CAD build for the part. Positions are in the model's coordinates, mm. Face numbers are marked on the shaded views. A direction names the side the tool comes from. Round coordinates to 2 decimals unless told otherwise and drop trailing zeros. Write each loop counter-clockwise with the first axis right and the second up, starting at its lowest first coordinate (ties: lowest second). Pieces come first, ordered by that corner, then holes. Notation, with made-up numbers: (26.25, -21.75) - (66.25, -21.75) arc R29 ccw to (66.25, 10.25) - close; hole circle Ø5 at (51.25, 4.25). An arc over 180 degrees is marked (long way). Answer in a Markdown table with one row per item.
Autodesk Inventor part; units mm, degrees
ref_plane "YZ Plane" through (0, 0, 0) normal (1, 0, 0) x (0, 1, 0)
ref_plane "XZ Plane" through (0, 0, 0) normal (0, 1, 0) x (-1, 0, 0)
ref_plane "XY Plane" through (0, 0, 0) normal (0, 0, 1) x (1, 0, 0)
sketch "Sketch1" plane through (0, 0, 0) normal (0, 1, 0) x (-1, 0, 0)
  line L0 (10.6592, 57.15) -> (-7.8828, 57.15)
  line L1 (-7.8828, 57.15) -> (-7.8828, -12.7)
  line L2 (-7.8828, -12.7) -> (10.6592, -12.7)
  line L3 (10.6592, 51.435) -> (-1.5328, 51.435)
  line L4 (-1.5328, 51.435) -> (-1.5328, 25.4)
  line L5 (-1.5328, 25.4) -> (10.6592, 25.4)
  line L6 (10.6592, 19.05) -> (-1.5328, 19.05)
  line L7 (-1.5328, 19.05) -> (-1.5328, -6.35)
  line L8 (-1.5328, -6.35) -> (10.6592, -6.35)
  line L9 (10.6592, -12.7) -> (10.6592, -6.35)
  line L10 (10.6592, 19.05) -> (10.6592, 25.4)
  line L11 (10.6592, 51.435) -> (10.6592, 57.15)
  point P0 (0, 0)
  dimension "d0" = 18.542
  dimension "d3" = 6.35
  dimension "d4" = 6.35
  dimension "d5" = 5.715
  dimension "d7" = 0
  dimension "d8" = 26.035
  dimension "d9" = 25.4
  dimension "d25" = 0
  dimension "d26" = 0
extrude "Extrusion1" add sketch "Sketch1" along normal blind 101.6
sketch "Sketch2" plane through (1.5328, 0, -6.35) normal (-1, 0, 0) x (0, 0, 1)
  line L0 (0, 0) -> (0, 101.6)
  line L1 (0, 0) -> (25.4, 0)
  point P0 (6.35, 0)
  point P1 (12.7, 25.4)
  point P2 (12.7, 50.8)
  point P3 (12.7, 76.2)
  dimension "d12" = 12.7
  dimension "d13" = 25.4
  dimension "d14" = 25.4
  dimension "d15" = 0
  dimension "d16" = 0
  dimension "d17" = 25.4
hole "Hole1" at (1.5328, 25.4, 6.35) at (1.5328, 50.8, 6.35) at (1.5328, 76.2, 6.35) direction (1, 0, 0) diameter 4.826 depth 25.4 tip angle 118
sketch "Sketch3" plane through (0, 101.6, 0) normal (0, 1, 0) x (1, 0, 0)
  line L0 (1.5328, -25.4) -> (-10.7917, -24.9696)
  line L1 (-10.7917, -24.9696) -> (-10.7917, -25.4)
  line L2 (-10.6592, -25.4) -> (1.5328, -25.4)
  line L3 (-10.7917, -25.4) -> (1.5328, -25.4)
  point P0 (0, 0)
  dimension "d27" = 2
extrude "Extrusion2" cut sketch "Sketch3" against normal blind 111.125
sketch "Sketch4" plane through (0, 101.6, 0) normal (0, 1, 0) x (1, 0, 0)
  line L0 (1.5328, -51.435) -> (-12.9577, -51.435)
  line L1 (-12.9577, -51.435) -> (-12.9577, -51.941)
  line L2 (-12.9577, -51.941) -> (1.5328, -51.435)
  point P0 (0, 0)
  dimension "d30" = 2
extrude "Extrusion3" cut sketch "Sketch4" against normal blind 119.0625
sketch "Sketch5" plane through (0, 101.6, 0) normal (0, 1, 0) x (1, 0, 0)
  line L0 (-10.6592, -57.15) -> (7.8828, -57.15)
  line L1 (7.8828, -57.15) -> (-13.0423, -56.4193)
  line L2 (-13.0423, -56.4193) -> (-13.0009, -57.15)
  line L3 (-13.0009, -57.15) -> (7.8828, -57.15)
  point P0 (0, 0)
  dimension "d33" = 2
extrude "Extrusion4" cut sketch "Sketch5" against normal blind 196.85
sketch "Sketch6" plane through (0, 101.6, 0) normal (0, 1, 0) x (1, 0, 0)
  line L0 (7.8828, 12.7) -> (-10.6592, 12.7)
  line L1 (7.8828, 12.7) -> (-16.8119, 12.7)
  line L2 (-16.8119, 12.7) -> (-16.8119, 11.8376)
  line L3 (7.8828, -57.15) -> (7.8828, 12.7)
  line L4 (-16.8119, 11.8376) -> (7.8828, 12.7)
  point P0 (0, 0)
  dimension "d36" = 2
extrude "Extrusion5" cut sketch "Sketch6" against normal blind 334.9625
sketch "Sketch7" plane through (1.5328, 0, 25.4) normal (-1, 0, 0) x (0, 0, 1)
  circle A0 centre (12.7901, 50.8553) radius 4.2212
  point P0 (-25.4, 0)
extrude "Extrusion6" cut sketch "Sketch7" against normal blind 58.7375
equation "\"d0\" = ElvDelWidth"
equation "\"d3\" = ElvDelFrontTabLength"
equation "\"d4\" = ElvDelMiddleTabLength"
equation "\"d9\" = ElvBeamWidth"
equation "\"d10\" = ElvDelHeight"
equation "\"ElvBeamWidth\" = 25.4"
equation "\"ElvDelWidth\" = 18.542"
equation "\"ElvDelHeight\" = 101.6"
equation "\"ElvDelFrontTabLength\" = 6.35"
equation "\"ElvDelDepth\" = 6.35"
equation "\"d2\" = ElvDelDepth"
equation "\"ElvCrossBeamLength\" = 304.8"
equation "\"ElvFixedBeamLength\" = 990.6"
equation "\"ElvMiddleBeamLength\" = 990.6"
equation "\"ElvFrontBeamLength\" = 990.6"
equation "\"ElvEndEffectLength\" = 431.8"
equation "\"ElvWallWidth\" = 1.5875"
equation "\"ElvTopBeamLength\" = 457.2"
equation "\"ElvHoleFromFront\" = 25.4"
equation "\"ElvHoleFromMid\" = 38.1"
equation "\"ElvHoleFromFixed\" = 50.8"
equation "\"ElvHoleFromBottom\" = 38.1"
equation "\"ElvRivetPlateLength\" = 76.2"
equation "\"ElvDelMiddleTabLength\" = 6.35"
properties part number "ElvDelV3" material "Acetal Resin, White"
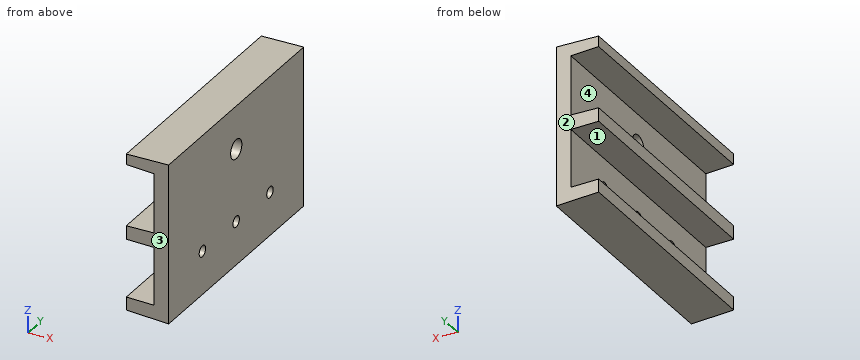
Q1. Saw through at D-D on x = 3.25. List the corners of the cut face in (y, z).
Computed:
| item | result |
|---|---|
| outline | (0, -12.54) - (101.6, -12.54) - (101.6, 56.99) - (0, 56.99) - close; hole circle Ø4.83 at (25.4, 6.35); hole circle Ø8.44 at (50.86, 38.19); hole circle Ø4.83 at (50.8, 6.35); hole circle Ø4.83 at (76.2, 6.35) |
Q2. Drill centre lines: line 1 (Y direction, x = 4.75, z = 6.35); line 2 (Z direction, x = 1.25, y = 61.5); line 3 (Z direction, x = -1.75, y = 50.5). Where is each one in solid material? Low to high.
Computed:
| item | result |
|---|---|
| line 1 | y = 0 to 22.99, 27.81 to 48.39, 53.21 to 73.79, 78.61 to 101.6 |
| line 2 | z = -12.47 to -6.35, 19.05 to 25.39, 51.44 to 56.92 |
| line 3 | z = -12.36 to -6.35, 19.05 to 25.29, 51.55 to 56.81 |
Q3. Pull direction Z, two halves, no side cores. Call the marked faces 3 and 4: released by +Z, released by -Z, zero draft, split by the parting line, or undercut.
Computed:
| item | result |
|---|---|
| face 3 | zero draft |
| face 4 | undercut |
Q4. Saw through at B-B on z = 6.35. List the corners of the cut face in (x, y), then the cut area to 3 significant figures.
Computed:
| item | result |
|---|---|
| outline | (1.53, 0) - (7.88, 0) - (7.88, 22.99) - (1.53, 22.99) - close; (1.53, 27.81) - (7.88, 27.81) - (7.88, 48.39) - (1.53, 48.39) - close; (1.53, 53.21) - (7.88, 53.21) - (7.88, 73.79) - (1.53, 73.79) - close; (1.53, 78.61) - (7.88, 78.61) - (7.88, 101.6) - (1.53, 101.6) - close |
| area | 553 mm2 |
Q5. 3-axis set-ups, long thin cutter, end or side, ignore diameter. For the marked faces 1 and 2: which of +Z, -Z, +X, -X, +Y, -Y reach the whole face in a straight line?
Computed:
| item | result |
|---|---|
| face 1 | -X, +Y, -Y |
| face 2 | +Z, -Z, +X, -X, +Y |
Q6. Flat gauge pins, fed straight in: pin 1 (1 mm diameter, centred on y = 46, z = 43, fed in from -X); pin 2 (5 mm diameter, centred on y = 50.86, z = 38.19, fed in from -X) (3 decimals); pin 3 (6 mm diameter, centred on x = -3.5, y = 43.5, fed in from +Z); pin 4 (2 mm diameter, centred on x = 1, y = 53, fed in from -Z). Where does each tip first touch, or does it go through?
Computed:
| item | result |
|---|---|
| pin 1 | stops at x = 1.53 |
| pin 2 | passes through |
| pin 3 | stops at z = 56.86 |
| pin 4 | stops at z = -12.49 |
Q7. Saw through at A-A on y = 25.4. List the corners of the cut face in (x, z) (3 decimals), then the cut area to 3 significant figures.
Computed:
| item | result |
|---|---|
| outline | (-10.659, -12.052) - (7.883, -12.7) - (7.883, 3.937) - (1.533, 3.937) - (1.533, -6.35) - (-10.659, -6.35) - close; (-10.659, 19.05) - (1.533, 19.05) - (1.533, 8.763) - (7.883, 8.763) - (7.883, 57.15) - (-10.659, 56.503) - (-10.659, 51.861) - (1.533, 51.435) - (1.533, 25.4) - (-10.659, 24.974) - close |
| area | 620 mm2 |
Q8. Saw through at C-C on x = -2. List the corners of the cut face in (y, z).
Computed:
| item | result |
|---|---|
| outline | (0, -12.35) - (101.6, -12.35) - (101.6, -6.35) - (0, -6.35) - close; (0, 19.05) - (101.6, 19.05) - (101.6, 25.28) - (0, 25.28) - close; (0, 51.56) - (101.6, 51.56) - (101.6, 56.8) - (0, 56.8) - close |
